Could you check a few things on this drawing? It's one solid part, dimensions in mm from its lowest x, y, z. A direction names the side the tool comes from. Coordinates: 2 decimals unless noted, no trailing zeros. Loops run counter-clockwise (first coordinate to the right, second up) from the corner with the lowest first, then second, coordinate; pieces in that order, holes last. Notation, with made-up numbers: (16.5, 21.25) -> (55.5, 21.25) arc R20 cw to (55.5, 42.25) -> close; hole circle Ø8 at (-4.5, -1.5). An arc over 180 degrees is marked (long way). One line per question, with ' | ' between items. Start each with the question number.
(1) Suppose I cut it at A-A (z = 9.25). Please give me the cut outline in (x, y), plus the area to 3 significant figures.
(2) Which directions (+Z, -Z, +X, -X, +Y, -Y) give clear straight access to the entire face, cutting with the end or side of a thin tool? Please do the marked faces 4 and 5.
(3) I'm going to push flat-ended pins straight in: pin 1 Ø1 at (x, y) = (2, 2) entering from -Z; pin 2 Ø1 at (x, y) = (8.5, 4.5) entering from +Z; pin 3 Ø3.5 at (x, z) = (4, 4.5) entering from -Y. Where does each tip first touch, or does it pass through?
(4) If I drill on line 1 along Z through (x, y) = (5, 1.35); line 2 along X through (y, z) = (3.15, 13.25); line 3 along Z through (x, y) = (6.75, 1.05) (1 decimal), over which ranges is the centre line in solid material (lowest first)?
(5) Suppose I cut it at C-C (y = 4.25). Please give me the cut outline in (x, z).
(6) If we mould it in two halves opening along X, with no side actions, what happens to the marked faces 1, 2 and 3? For each: pulls with the +X half, pulls with the -X half, needs draft (parallel to the pull), parting line crosses it, or undercut.
(7) Suppose I cut it at D-D (y = 1.75). Please give me the cut outline in (x, z).
(8) Suppose I cut it at B-B (x = 5). Please give me the cut outline in (y, z).
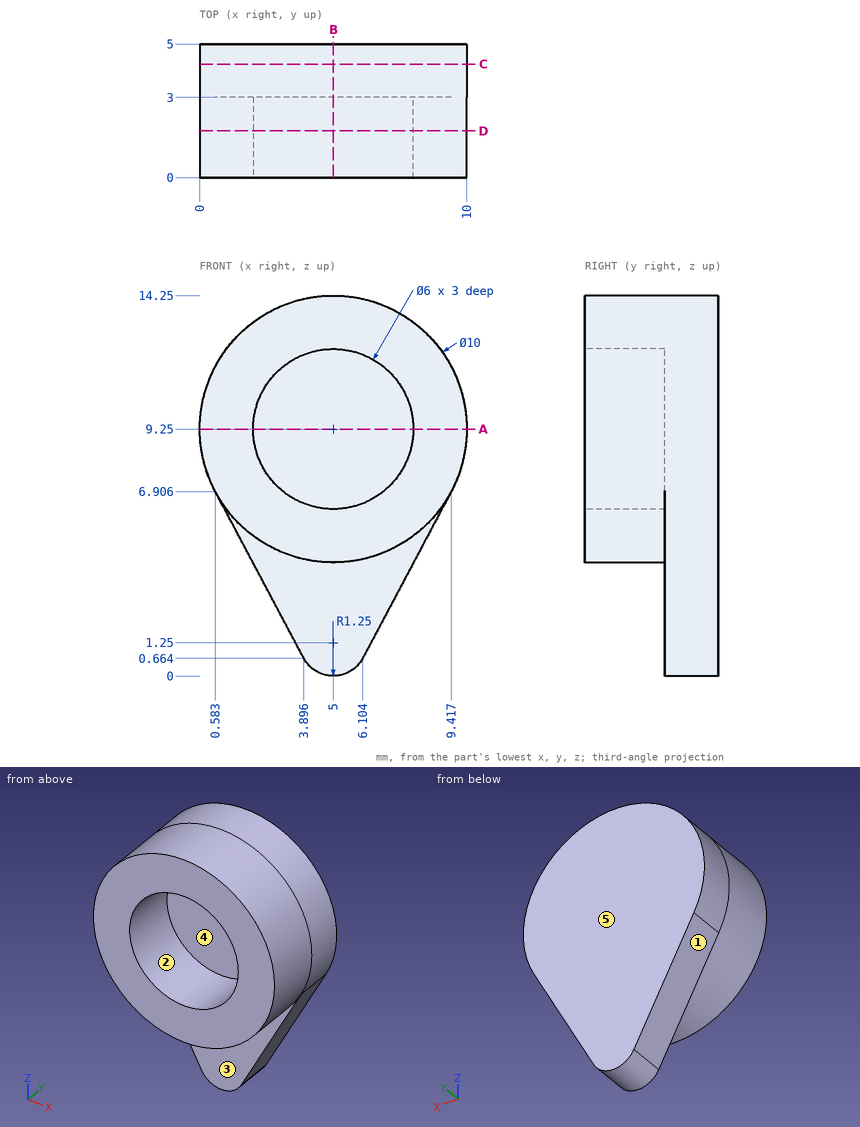
Checks:
1) outline: (0, 0) -> (2, 0) -> (2, 3) -> (8, 3) -> (8, 0) -> (10, 0) -> (10, 5) -> (0, 5) -> close | area: 32.0 mm^2
2) face 4: -Y | face 5: +Z, -Z, +X, -X, +Y
3) pin 1: stops at z = 4.92 | pin 2: stops at z = 13.25 | pin 3: stops at y = 0
4) line 1: z = 4.25 to 6.25, 12.25 to 14.25 | line 2: x = 2 to 8 | line 3: z = 4.6 to 6.8, 11.7 to 13.9
5) outline: (0.58, 6.91) -> (3.9, 0.66) arc R1.25 ccw to (6.1, 0.66) -> (9.42, 6.91) arc R5 ccw (long way) to start
6) face 1: pulls with the -X half | face 2: undercut | face 3: needs draft
7) outline: circle Ø10 at (5, 9.25); hole circle Ø6 at (5, 9.25)
8) outline: (0, 4.25) -> (3, 4.25) -> (3, 0) -> (5, 0) -> (5, 14.25) -> (0, 14.25) -> (0, 12.25) -> (3, 12.25) -> (3, 6.25) -> (0, 6.25) -> close
